Work out the finished part from the listing and answer in its coordinate system (mm). A direction names the side the tool comes from. Coordinates: 2 decimals unless noted, no trailing zeros. Loops run counter-clockwise (first coordinate to the right, second up) from the corner with the lowest first, then second, coordinate; pieces in that order, holes last. Notation, with made-up numbers: (40.5, 59) -> (93.5, 59) arc R9 ccw to (93.5, 65) -> close; hole circle Ø10 at (-39.5, -35.75). An arc over 180 degrees is marked (long way). Answer as CSV lines item,"result".
```python
from build123d import *

# Parameters (mm, degrees)
F1_DEPTH = 254
F2_R     = 9.165436
F2_R_2   = 7.9375
F3_DEPTH = 101.6
F4_R     = 9.165436
F4_R_2   = 7.9375
F5_DEPTH = 101.6
F6_R     = 3.175
F7_DEPTH = 25.4
F8_R     = 3.175
F9_DEPTH = 25.4


with BuildPart() as f1:
    # F0 (on Top) → F1 (new body)
    with BuildSketch(Plane.XY):
        Polygon((-4.582718, 7.9375), (-9.165436, 0), (-4.582718, -7.9375), (4.582718, -7.9375), (9.165436, 0), (4.582718, 7.9375), align=None)
    extrude(amount=F1_DEPTH)

    # F2 (on face) → F3 (cut)
    with BuildSketch(Plane.XY.offset(254)):
        Circle(F2_R)
        Circle(F2_R_2, mode=Mode.SUBTRACT)
    extrude(amount=-F3_DEPTH, mode=Mode.SUBTRACT)

    # F4 (on face) → F5 (cut)
    with BuildSketch(Plane(origin=(0, 0, 0), x_dir=(1, 0, 0), z_dir=(0, 0, -1))):
        Circle(F4_R)
        Circle(F4_R_2, mode=Mode.SUBTRACT)
    extrude(amount=-F5_DEPTH, mode=Mode.SUBTRACT)

    # F6 (on face) → F7 (cut)
    with BuildSketch(Plane(origin=(0, 0, 0), x_dir=(1, 0, 0), z_dir=(0, 0, -1))):
        Circle(F6_R)
    extrude(amount=-F7_DEPTH, mode=Mode.SUBTRACT)

    # F8 (on face) → F9 (cut)
    with BuildSketch(Plane.XY.offset(254)):
        Circle(F8_R)
    extrude(amount=-F9_DEPTH, mode=Mode.SUBTRACT)


solid = f1.part
```
(1) Flat-ended cylindrical pins translate along their axes: pin 1 Ø0.7 at (x, y) = (7.5, 2) entering from -Z; pin 2 Ø1 at (x, z) = (1.5, 98) entering from -Y; pin 3 Ø3 at (x, z) = (3, 32) entering from -Y; pin 4 Ø3 at (x, y) = (-1, -1) entering from -Z. Find the tip coordinate at first contact, or state that the pin passes through.
Computed values:
pin 1,"z = 0"
pin 2,"y = -7.87"
pin 3,"y = -7.79"
pin 4,"z = 25.4"
(2) A cutting plane is placed at A-A, the plane z = 119. Write down the section's boundary in (x, y).
Computed values:
outline,"(-9.17, 0) -> (-4.58, -7.94) -> (4.58, -7.94) -> (9.17, 0) -> (4.58, 7.94) -> (-4.58, 7.94) -> close"
(3) Which of the six approach directions +Z, -Z, +X, -X, +Y, -Y give full straight-line access (tool end or side, diameter ignored) to faces 5 (the face through (-4, -7.1, 152.4)), 6 (the face through (4.2, -7.1, 101.6)), 7 (the face through (0, 0, 25.4))?
Computed values:
face 5,"+Z, -X, -Y"
face 6,"-Z, +X, -Y"
face 7,"-Z"
(4) Consider line 1 along Y through (x, z) = (0, 15.5) (1 decimal); line 2 along Y through (x, z) = (0.5, 93). Determine where each line is inside the solid, lowest interval first.
Computed values:
line 1,"-7.9 to -3.2, 3.2 to 7.9"
line 2,"-7.92 to 7.92"
(5) For a pull along Y with two mould halves and no side action, classify faces 1 (the face through (0, 0, 228.6)), 2 (the face through (-0.69, 3.1, 12.52)), 3 (the face through (6.842, -4.024, 126.644)), 4 (the face through (4.2, 7.1, 101.6)) as pulls with the +Y half, pulls with the -Y half, needs draft (parallel to the pull), parting line crosses it, or undercut.
Computed values:
face 1,"undercut"
face 2,"undercut"
face 3,"pulls with the -Y half"
face 4,"needs draft"
